from build123d import *

# Parameters (mm, degrees)
SALIENTE_EXTRUIR1_DEPTH = 4
CROQUIS2_R              = 1.5
CORTAR_EXTRUIR1_DEPTH   = 13
CROQUIS3_R              = 1.5
CORTAR_EXTRUIR2_DEPTH   = 23


with BuildPart() as part:
    # Croquis1 → Saliente-Extruir1 (new body)
    with BuildSketch(Plane(origin=(0, 0, 0), x_dir=(0, 0, -1), z_dir=(1, 0, 0))):
        Polygon((31.77750931, 8.602977891), (79.291659343, 76.856040613), (110.141305144, 76.856040613), (81.77750931, 8.602977891), (81.77750931, -11.397022109), (31.77750931, -11.397022109), align=None)
    extrude(amount=SALIENTE_EXTRUIR1_DEPTH)

    # Croquis2 → Cortar-Extruir1 (cut)
    with BuildSketch(Plane(origin=(4, 0, 0), x_dir=(0, 0, -1), z_dir=(1, 0, 0))):
        with Locations((84.214840877, 71.856040613)):
            Circle(CROQUIS2_R)
        with Locations((101.452703983, 71.856040613)):
            Circle(CROQUIS2_R)
    extrude(amount=-CORTAR_EXTRUIR1_DEPTH, mode=Mode.SUBTRACT)

    # Croquis3 → Cortar-Extruir2 (cut)
    with BuildSketch(Plane.ZY):
        with Locations((-66.77750931, -1.397022109)):
            Circle(CROQUIS3_R)
        with Locations((-46.77750931, -1.397022109)):
            Circle(CROQUIS3_R)
    extrude(amount=-CORTAR_EXTRUIR2_DEPTH, mode=Mode.SUBTRACT)


solid = part.part
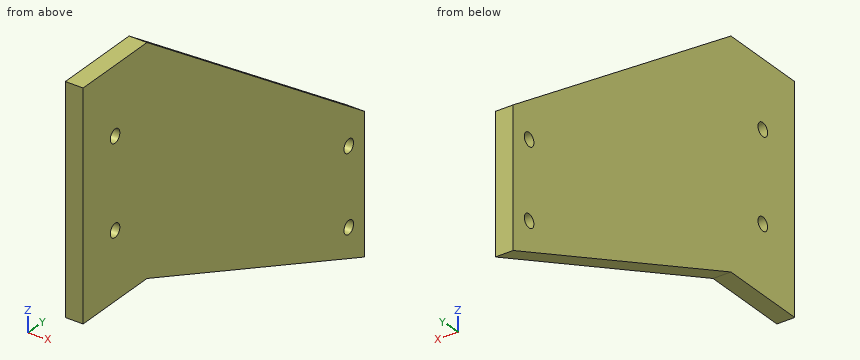
Geometry check sheet. Reference: the model listing, model coordinates, mm. Give positions to 0.01 mm unless a question says otherwise; leave off trailing zeros. Loops run counter-clockwise (first coordinate to the right, second up) from the corner with the lowest first, then second, coordinate; pieces in that order, holes last. Notation, with made-up numbers: M 83,55 L 87,55 A23 ccw 87,74 Z; hole C 27.5,45 d4. An arc over 180 degrees is marked long. Answer as a JSON object with one key per item and string values. Group by question number.
Item 1: Sectioned sample at C-C on z = -43. Record the boundary of the cut face in (x, y), plus the area to 3 significant figures.
Item 2: Sectioned sample at B-B on y = 6. Record the boundary of the cut face in (x, z).
Item 3: Material ranges on L1, parallel to Z at x = 0.8, y = 4; L2, parallel to Z at x = 2.6, y = -2.5; L3, parallel to Y at x = 2.5, z = -101, recorded low to high.
Item 4: Sectioned sample at A-A on x = 1.35. Record the boundary of the cut face in (y, z), plus the area to 3 significant figures.
Item 5: Gauge pin test, flat end, axial feed: pin 1 (1.5 mm diameter, centred on x = 3, y = -1, fed in from -Z). Record the tip position at first contact, or that the pin passes through.
Findings below:
{
 "1": {"outline": "M 0,-11.4 L 4,-11.4 L 4,24.72 L 0,24.72 Z", "area": "144 mm2"},
 "2": {"outline": "M 0,-81.78 L 4,-81.78 L 4,-31.78 L 0,-31.78 Z"},
 "3": {"L1": "-81.78 to -31.78", "L2": "-81.78 to -67.79, -65.76 to -47.79, -45.76 to -31.78", "L3": "54.86 to 70.43, 73.29 to 76.86"},
 "4": {"outline": "M -11.4,-81.78 L 8.6,-81.78 L 76.86,-110.14 L 76.86,-79.29 L 8.6,-31.78 L -11.4,-31.78 Z; hole C -1.4,-66.78 d3; hole C -1.4,-46.78 d3; hole C 71.86,-101.45 d3; hole C 71.86,-84.21 d3", "area": "3,730 mm2"},
 "5": {"pin 1": "z = -81.78"}
}
